Geometry check sheet. Reference: the model listing, model coordinates, mm. Face numbers are marked on the shaded views. Round coordinates to 2 decimals unless told otherwise and drop trailing zeros. Order: outer loops, then holes, each group sorted by start corner. A loop starts at its lowest first (then second) coordinate and runs counter-clockwise, first axis right, second up.
(1) Draft check along X on the marked faces 1 and 2. Enter one of: pulls with the +X half, pulls with the -X half, needs draft (parallel to the pull), parting line crosses it, or undercut.
(2) Thickness scan on L1, parallel to X at y = -1.75, z = -3.75; L2, parallel to Y at x = 5, z = 1.5. Record the ranges inside material, lowest first.
(3) Gauge pin test, flat ends, axial feed: P1, Ø5, axis at x = 34, y = -0.5, coming from the -Z side; P2, Ø4, axis at y = 2, z = -3.5, coming from the -X side; P3, Ø1.5, axis at x = 21, y = -1.5, coming from the -Z side. Record the tip position at first contact, or that the pin passes through.
(4) Cross-section at A-A on x = 38.5. Enter the section's corners in (y, z), and give its area (3 significant figures).
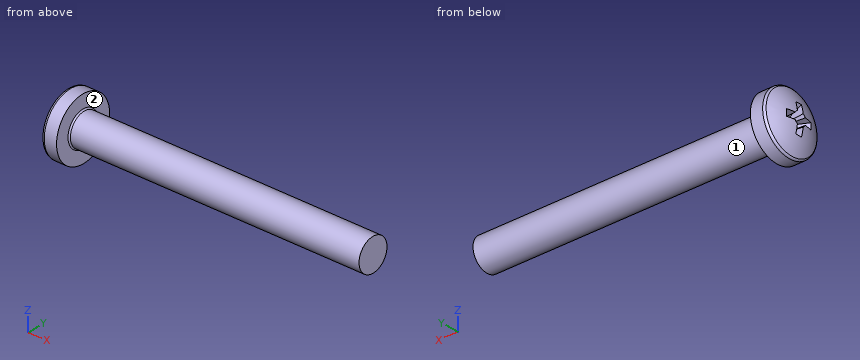
from build123d import *

# Parameters (mm, degrees)
RECPAT_COUNT = 2
RECPAT_ANGLE = 90


with BuildPart() as part:
    # Fillet1: read off the stored shape, not the designer's step
    # Fillet1 outline → Fillet1 (revolve)
    with BuildSketch(Plane.YX):
        with BuildLine():
            Line((2.5, 3.9), (2.5, 48.7))
            Line((2.5, 48.7), (0, 48.7))
            Line((0, 48.7), (0, 0))
            ThreePointArc((0, 0), (2.386856711, 0.364365446), (4.556291394, 1.42427124))
            ThreePointArc((4.556291394, 1.42427124), (4.698642149, 1.58538712), (4.75, 1.79415598))
            Line((4.75, 1.79415598), (4.75, 3.7))
            Line((4.75, 3.7), (2.7, 3.7))
            ThreePointArc((2.7, 3.7), (2.558578644, 3.758578644), (2.5, 3.9))
        make_face()
    revolve(axis=Axis((0, 0, 0), (1, 0, 0)))

    # Sketch3 → Recess section 0
    with BuildSketch(Plane(origin=(0, 0, 0), x_dir=(0, 0, -1), z_dir=(1, 0, 0))):
        with BuildLine():
            Line((0.515, -2.35), (-0.515, -2.35))
            Line((-0.515, -2.35), (-0.515, 2.35))
            Line((-0.515, 2.35), (0.515, 2.35))
            Line((0.515, 2.35), (0.515, -2.35))
        make_face()
    # Sketch4 → Recess section 1
    with BuildSketch(Plane(origin=(2.74, 0, 0), x_dir=(0, 0, -1), z_dir=(1, 0, 0))):
        with BuildLine():
            Line((0.515, -0.983886622), (-0.515, -0.983886622))
            Line((-0.515, -0.983886622), (-0.515, 0.983886622))
            Line((-0.515, 0.983886622), (0.515, 0.983886622))
            Line((0.515, 0.983886622), (0.515, -0.983886622))
        make_face()
    recess = loft(mode=Mode.SUBTRACT)

    # RecPat: Recess ×2 about axis
    recpat_axis = Axis((0, 0, 0), (1, 0, 0))
    for i in range(1, RECPAT_COUNT):
        add(recess.rotate(recpat_axis, i * RECPAT_ANGLE / (RECPAT_COUNT - 1)), mode=Mode.SUBTRACT)

    # RecCorSke → RecessCore (revolve, cut)
    with BuildSketch(Plane.XY, mode=Mode.PRIVATE) as recesscore_sk:
        Polygon((0, 0), (0, 1.042599465), (2.74, 0.851), (3.016506661, 0), align=None)
    revolve(recesscore_sk.sketch.rotate(Axis((-3.175, 0, 0), (1, 0, 0)), 90), axis=Axis((-3.175, 0, 0), (1, 0, 0)), mode=Mode.SUBTRACT)


solid = part.part
Found:
1. face 1: needs draft
1. face 2: pulls with the +X half
2. L1: x = 1.15 to 3.7
2. L2: y = -2 to 2
3. P1: stops at z = -2.5
3. P2: stops at x = 0.26
3. P3: stops at z = -2.38
4. outline: circle Ø5 at (0, 0)
4. area: 19.6 mm2
